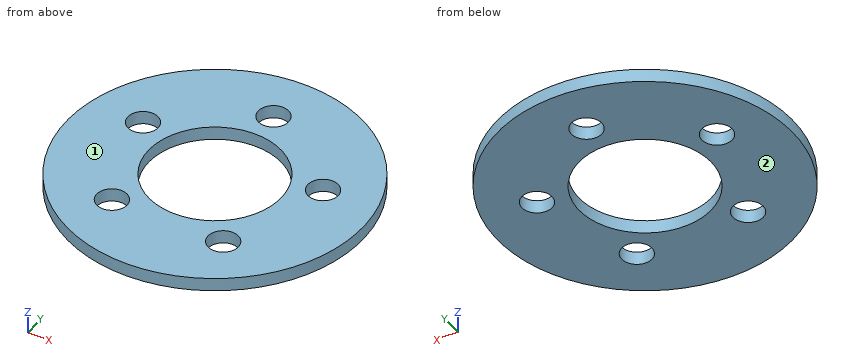
from build123d import *

# Parameters (mm, degrees)
SKETCH3_R           = 17.78
SKETCH3_R_2         = 7.9629
SKETCH3_R_3         = 1.8288
BOSS_EXTRUDE2_DEPTH = 1.5875


with BuildPart() as part:
    # Sketch3 → Boss-Extrude2 (new body)
    with BuildSketch(Plane(origin=(0, 0, -15.875), x_dir=(-1, 0, 0), z_dir=(0, 0, -1))):
        Circle(SKETCH3_R)
        Circle(SKETCH3_R_2, mode=Mode.SUBTRACT)
        with Locations((-6.759530401, -9.303695435)):
            Circle(SKETCH3_R_3, mode=Mode.SUBTRACT)
        with Locations((6.759530401, -9.303695435)):
            Circle(SKETCH3_R_3, mode=Mode.SUBTRACT)
        with Locations((10.937149937, 3.553695435)):
            Circle(SKETCH3_R_3, mode=Mode.SUBTRACT)
        with Locations((0, 11.5)):
            Circle(SKETCH3_R_3, mode=Mode.SUBTRACT)
        with Locations((-10.937149937, 3.553695435)):
            Circle(SKETCH3_R_3, mode=Mode.SUBTRACT)
    extrude(amount=BOSS_EXTRUDE2_DEPTH)


solid = part.part
Design review of the part built by this model. Coordinates are the model's own, in mm. Face numbers are marked on the shaded views. Give positions to 0.01 mm unless a question says otherwise; leave off trailing zeros. Write each loop counter-clockwise with the first axis right and the second up, starting at its lowest first coordinate (ties: lowest second). Pieces come first, ordered by that corner, then holes. Notation, with made-up numbers: M 82.5,-33 L 104.5,-33 A15 cw 104.5,-18 Z; hole C 89,15.5 d4. An arc over 180 degrees is marked long. Answer as a JSON object with one key per item and string values. Group by question number.
1) We need section A-A (y = 0). Give the boundary of the cut face in (x, z) (1 decimal).
2) Mouldability with a two-part tool opening along Z and no side actions: class the marked faces 1 and 2 as released by +Z, released by -Z, zero draft, split by the parting line, or undercut.
3) For line 1 along Y through (x, z) = (0, -17); line 2 along Y through (x, z) = (-7, -17.2); line 3 along X through (y, z) = (-8, -17.25), list the stretches that pass through material, from the lowest coordinate up.
4) We need section B-B (x = 1). Give the boundary of the cut face in (y, z) (1 decimal), and give its area (3 significant figures).
5) We need section D-D (z = -16.15). Give the boundary of the cut face in (x, y), and give its area (3 significant figures).
6) We need section C-C (x = -3.5). Give the boundary of the cut face in (y, z) (1 decimal), and give its area (3 significant figures).
Answer key:
{
 "1": {"outline": "M -17.8,-17.5 L -8,-17.5 L -8,-15.9 L -17.8,-15.9 Z; M 8,-17.5 L 17.8,-17.5 L 17.8,-15.9 L 8,-15.9 Z"},
 "2": {"face 1": "released by +Z", "face 2": "released by -Z"},
 "3": {"line 1": "y = -17.78 to -7.96, 7.96 to 9.67, 13.33 to 17.78", "line 2": "y = -16.34 to -11.12, -7.49 to -3.8, 3.8 to 16.34", "line 3": "x = -15.88 to -8.04, -5.48 to 5.48, 8.04 to 15.88"},
 "4": {"outline": "M -17.8,-17.5 L -7.9,-17.5 L -7.9,-15.9 L -17.8,-15.9 Z; M 7.9,-17.5 L 10,-17.5 L 10,-15.9 L 7.9,-15.9 Z; M 13,-17.5 L 17.8,-17.5 L 17.8,-15.9 L 13,-15.9 Z", "area": "26.4 mm²"},
 "5": {"outline": "C 0,0 d35.56; hole C -10.94,3.55 d3.66; hole C -6.76,-9.3 d3.66; hole C 0,0 d15.93; hole C 0,11.5 d3.66; hole C 6.76,-9.3 d3.66; hole C 10.94,3.55 d3.66", "area": "741 mm²"},
 "6": {"outline": "M -17.4,-17.5 L -7.2,-17.5 L -7.2,-15.9 L -17.4,-15.9 Z; M 7.2,-17.5 L 17.4,-17.5 L 17.4,-15.9 L 7.2,-15.9 Z", "area": "32.6 mm²"}
}
